from build123d import *

# Parameters (mm, degrees)
PAROI_DEPTH                    = 55
ESQUISSE11_W                   = 10
ESQUISSE11_H                   = 10
FIXATION_PAROI_BASE_DEPTH      = 3
ESQUISSE13_R                   = 1.5
TROU_FIXATION_PAROI_BASE_DEPTH = 4
EXTRUSION_BUMPER_REACH         = 108.066
ESQUISSE14_W                   = 172.132034356
ESQUISSE14_H                   = 30
BOSS_EXTRU_1_REACH             = 108.066
ESQUISSE15_W                   = 20
ESQUISSE15_H                   = 5
BOSS_EXTRU_2_DEPTH             = 35
ENL_V_MAT_EXTRU_1_REACH        = 108.066
ESQUISSE17_R                   = 2
ESQUISSE18_W                   = 10
ESQUISSE18_H                   = 10
ESQUISSE18_R                   = 1.5
BOSS_EXTRU_3_DEPTH             = 3
ESQUISSE20_W                   = 10
ESQUISSE20_H                   = 6
ESQUISSE20_W_2                 = 6
ESQUISSE20_H_2                 = 8
ENL_V_MAT_EXTRU_2_DEPTH        = 107.066017178
BOSS_EXTRU_4_DEPTH             = 5
BOSS_EXTRU_5_DEPTH             = 5
ENL_V_MAT_EXTRU_3_REACH        = 83.632
ESQUISSE25_R                   = 1.5
ESQUISSE35_R                   = 3
ENL_V_MAT_EXTRU_4_DEPTH        = 12
CONG_1_R                       = 5
CONG_2_R                       = 2


with BuildPart() as part:
    # Esquisse1 → paroi (new body)
    with BuildSketch(Plane.XY):
        with BuildLine():
            Line((0, 150), (0, 145))
            ThreePointArc((0, 145), (102.530483272, 102.530483272), (145, 0))
            Line((145, 0), (150, 0))
            ThreePointArc((150, 0), (106.066017178, 106.066017178), (0, 150))
        make_face()
    extrude(amount=PAROI_DEPTH)

    # Esquisse11 → fixation_paroi_base (add)
    with BuildSketch(Plane(origin=(0, 0, 0), x_dir=(-1, 0, 0), z_dir=(0, 0, -1))):
        with Locations((-140, 5)):
            Rectangle(ESQUISSE11_W, ESQUISSE11_H)
        with Locations((-5, 140)):
            Rectangle(ESQUISSE11_W, ESQUISSE11_H)
    extrude(amount=-FIXATION_PAROI_BASE_DEPTH)

    # Esquisse13 → trou_fixation_paroi_base (cut, through all)
    with BuildSketch(Plane.XY.offset(3)):
        with Locations((5, 140)):
            Circle(ESQUISSE13_R)
        with Locations((140, 5)):
            Circle(ESQUISSE13_R)
    extrude(amount=-TROU_FIXATION_PAROI_BASE_DEPTH, mode=Mode.SUBTRACT)

    # Esquisse14 → extrusion bumper (cut, up to next)
    with BuildSketch(Plane(origin=(75, 75, 0), x_dir=(-0.707106781, 0.707106781, 0), z_dir=(-0.707106781, -0.707106781, 0)), mode=Mode.PRIVATE) as extrusion_bumper_sk1:
        with Locations((0, -25)):
            Rectangle(ESQUISSE14_W, ESQUISSE14_H)
    extrusion_bumper_tool1 = extrude(extrusion_bumper_sk1.sketch, amount=-EXTRUSION_BUMPER_REACH, mode=Mode.PRIVATE) & part.part
    add(extrusion_bumper_tool1.solids().sort_by_distance((75, 75, 25))[0], mode=Mode.SUBTRACT)

    # Esquisse15 → Boss.-Extru.1 (add, up to next)
    with BuildSketch(Plane(origin=(75, 75, 0), x_dir=(-0.707106781, 0.707106781, 0), z_dir=(-0.707106781, -0.707106781, 0)), mode=Mode.PRIVATE) as boss_extru_1_sk1:
        with Locations((76.066017178, -42.5)):
            Rectangle(ESQUISSE15_W, ESQUISSE15_H)
    boss_extru_1_tool1 = extrude(boss_extru_1_sk1.sketch, amount=-BOSS_EXTRU_1_REACH, mode=Mode.PRIVATE) - part.part
    add(boss_extru_1_tool1.solids().sort_by_distance((21.213203, 128.786797, 42.5))[0])
    # Esquisse15 → Boss.-Extru.1 (add, up to next)
    with BuildSketch(Plane(origin=(75, 75, 0), x_dir=(-0.707106781, 0.707106781, 0), z_dir=(-0.707106781, -0.707106781, 0)), mode=Mode.PRIVATE) as boss_extru_1_sk2:
        with Locations((-76.066017178, -42.5)):
            Rectangle(ESQUISSE15_W, ESQUISSE15_H)
    boss_extru_1_tool2 = extrude(boss_extru_1_sk2.sketch, amount=-BOSS_EXTRU_1_REACH, mode=Mode.PRIVATE) - part.part
    add(boss_extru_1_tool2.solids().sort_by_distance((128.786797, 21.213203, 42.5))[0])
    # Esquisse15 → Boss.-Extru.1 (add, up to next)
    with BuildSketch(Plane(origin=(75, 75, 0), x_dir=(-0.707106781, 0.707106781, 0), z_dir=(-0.707106781, -0.707106781, 0)), mode=Mode.PRIVATE) as boss_extru_1_sk3:
        with Locations((76.066017178, -7.5)):
            Rectangle(ESQUISSE15_W, ESQUISSE15_H)
    boss_extru_1_tool3 = extrude(boss_extru_1_sk3.sketch, amount=-BOSS_EXTRU_1_REACH, mode=Mode.PRIVATE) - part.part
    add(boss_extru_1_tool3.solids().sort_by_distance((21.213203, 128.786797, 7.5))[0])
    # Esquisse15 → Boss.-Extru.1 (add, up to next)
    with BuildSketch(Plane(origin=(75, 75, 0), x_dir=(-0.707106781, 0.707106781, 0), z_dir=(-0.707106781, -0.707106781, 0)), mode=Mode.PRIVATE) as boss_extru_1_sk4:
        with Locations((-76.066017178, -7.5)):
            Rectangle(ESQUISSE15_W, ESQUISSE15_H)
    boss_extru_1_tool4 = extrude(boss_extru_1_sk4.sketch, amount=-BOSS_EXTRU_1_REACH, mode=Mode.PRIVATE) - part.part
    add(boss_extru_1_tool4.solids().sort_by_distance((128.786797, 21.213203, 7.5))[0])

    # Esquisse16 → Boss.-Extru.2 (add)
    with BuildSketch(Plane.XY.offset(45)):
        Polygon((135.857864376, 14.142135624), (121.715728753, 28.284271247), (125.251262658, 31.819805153), (139.393398282, 17.67766953), align=None)
        Polygon((28.284271247, 121.715728753), (14.142135624, 135.857864376), (17.67766953, 139.393398282), (31.819805153, 125.251262658), align=None)
    extrude(amount=-BOSS_EXTRU_2_DEPTH)

    # Esquisse17 → Enlèv. mat.-Extru.1 (cut, up to next)
    with BuildSketch(Plane(origin=(75, 75, 0), x_dir=(-0.707106781, 0.707106781, 0), z_dir=(-0.707106781, -0.707106781, 0)), mode=Mode.PRIVATE) as enl_v_mat_extru_1_sk1:
        with Locations((76.066017178, -25)):
            Circle(ESQUISSE17_R)
    enl_v_mat_extru_1_tool1 = extrude(enl_v_mat_extru_1_sk1.sketch, amount=-ENL_V_MAT_EXTRU_1_REACH, mode=Mode.PRIVATE) & part.part
    add(enl_v_mat_extru_1_tool1.solids().sort_by_distance((21.213203, 128.786797, 25))[0], mode=Mode.SUBTRACT)
    # Esquisse17 → Enlèv. mat.-Extru.1 (cut, up to next)
    with BuildSketch(Plane(origin=(75, 75, 0), x_dir=(-0.707106781, 0.707106781, 0), z_dir=(-0.707106781, -0.707106781, 0)), mode=Mode.PRIVATE) as enl_v_mat_extru_1_sk2:
        with Locations((-76.066017178, -25)):
            Circle(ESQUISSE17_R)
    enl_v_mat_extru_1_tool2 = extrude(enl_v_mat_extru_1_sk2.sketch, amount=-ENL_V_MAT_EXTRU_1_REACH, mode=Mode.PRIVATE) & part.part
    add(enl_v_mat_extru_1_tool2.solids().sort_by_distance((128.786797, 21.213203, 25))[0], mode=Mode.SUBTRACT)

    # Esquisse18 → Boss.-Extru.3 (add)
    with BuildSketch(Plane.XY.offset(55)):
        with Locations((5, 140)):
            Rectangle(ESQUISSE18_W, ESQUISSE18_H)
        with Locations((5, 140)):
            Circle(ESQUISSE18_R, mode=Mode.SUBTRACT)
        with Locations((140, 5)):
            Rectangle(ESQUISSE18_W, ESQUISSE18_H)
        with Locations((140, 5)):
            Circle(ESQUISSE18_R, mode=Mode.SUBTRACT)
    extrude(amount=-BOSS_EXTRU_3_DEPTH)

    # Esquisse20 → Enlèv. mat.-Extru.2 (cut, through all)
    with BuildSketch(Plane(origin=(75, 75, 0), x_dir=(-0.707106781, 0.707106781, 0), z_dir=(-0.707106781, -0.707106781, 0))):
        with Locations((76.066017178, -34)):
            Rectangle(ESQUISSE20_W, ESQUISSE20_H)
        with Locations((76.066017178, -16)):
            Rectangle(ESQUISSE20_W_2, ESQUISSE20_H_2)
        with Locations((-76.066017178, -34)):
            Rectangle(ESQUISSE20_W, ESQUISSE20_H)
        with Locations((-76.066017178, -16)):
            Rectangle(ESQUISSE20_W_2, ESQUISSE20_H_2)
    extrude(amount=-ENL_V_MAT_EXTRU_2_DEPTH, mode=Mode.SUBTRACT)

    # Esquisse21 → Boss.-Extru.4 (add)
    with BuildSketch(Plane.XY.offset(45)):
        Polygon((71.4177849, 130.81475452), (78.488852712, 123.743686708), (69.650017947, 114.904851943), (62.578950135, 121.975919755), align=None)
        Polygon((130.81475452, 71.4177849), (123.743686708, 78.488852712), (114.904851943, 69.650017947), (121.975919755, 62.578950135), align=None)
    extrude(amount=-BOSS_EXTRU_4_DEPTH)

    # Esquisse24 → Boss.-Extru.5 (add)
    with BuildSketch(Plane.XY.offset(10)):
        Polygon((62.578950135, 121.975919755), (71.065878403, 130.462848023), (78.136946215, 123.391780211), (69.650017947, 114.904851943), align=None)
        Polygon((121.975919755, 62.578950135), (130.462848023, 71.065878403), (123.391780211, 78.136946215), (114.904851943, 69.650017947), align=None)
    extrude(amount=-BOSS_EXTRU_5_DEPTH)

    # Esquisse25 → Enlèv. mat.-Extru.3 (cut, up to next)
    with BuildSketch(Plane(origin=(92.277434945, 92.277434945, 0), x_dir=(0, 0, 1), z_dir=(-0.707106781, -0.707106781, 0)), mode=Mode.PRIVATE) as enl_v_mat_extru_3_sk1:
        with Locations((42.5, 37.5)):
            Circle(ESQUISSE25_R)
    enl_v_mat_extru_3_tool1 = extrude(enl_v_mat_extru_3_sk1.sketch, amount=-ENL_V_MAT_EXTRU_3_REACH, mode=Mode.PRIVATE) & part.part
    add(enl_v_mat_extru_3_tool1.solids().sort_by_distance((65.760931, 118.793939, 42.5))[0], mode=Mode.SUBTRACT)
    # Esquisse25 → Enlèv. mat.-Extru.3 (cut, up to next)
    with BuildSketch(Plane(origin=(92.277434945, 92.277434945, 0), x_dir=(0, 0, 1), z_dir=(-0.707106781, -0.707106781, 0)), mode=Mode.PRIVATE) as enl_v_mat_extru_3_sk2:
        with Locations((42.5, -37.5)):
            Circle(ESQUISSE25_R)
    enl_v_mat_extru_3_tool2 = extrude(enl_v_mat_extru_3_sk2.sketch, amount=-ENL_V_MAT_EXTRU_3_REACH, mode=Mode.PRIVATE) & part.part
    add(enl_v_mat_extru_3_tool2.solids().sort_by_distance((118.793939, 65.760931, 42.5))[0], mode=Mode.SUBTRACT)
    # Esquisse25 → Enlèv. mat.-Extru.3 (cut, up to next)
    with BuildSketch(Plane(origin=(92.277434945, 92.277434945, 0), x_dir=(0, 0, 1), z_dir=(-0.707106781, -0.707106781, 0)), mode=Mode.PRIVATE) as enl_v_mat_extru_3_sk3:
        with Locations((7.5, 37.5)):
            Circle(ESQUISSE25_R)
    enl_v_mat_extru_3_tool3 = extrude(enl_v_mat_extru_3_sk3.sketch, amount=-ENL_V_MAT_EXTRU_3_REACH, mode=Mode.PRIVATE) & part.part
    add(enl_v_mat_extru_3_tool3.solids().sort_by_distance((65.760931, 118.793939, 7.5))[0], mode=Mode.SUBTRACT)
    # Esquisse25 → Enlèv. mat.-Extru.3 (cut, up to next)
    with BuildSketch(Plane(origin=(92.277434945, 92.277434945, 0), x_dir=(0, 0, 1), z_dir=(-0.707106781, -0.707106781, 0)), mode=Mode.PRIVATE) as enl_v_mat_extru_3_sk4:
        with Locations((7.5, -37.5)):
            Circle(ESQUISSE25_R)
    enl_v_mat_extru_3_tool4 = extrude(enl_v_mat_extru_3_sk4.sketch, amount=-ENL_V_MAT_EXTRU_3_REACH, mode=Mode.PRIVATE) & part.part
    add(enl_v_mat_extru_3_tool4.solids().sort_by_distance((118.793939, 65.760931, 7.5))[0], mode=Mode.SUBTRACT)

    # Esquisse35 → Enlèv. mat.-Extru.4 (cut)
    with BuildSketch(Plane(origin=(106.066017178, 106.066017178, 0), x_dir=(0, 0, 1), z_dir=(-0.707106781, -0.707106781, 0))):
        with Locations((42.5, -37.5)):
            Circle(ESQUISSE35_R)
        with Locations((42.5, 37.5)):
            Circle(ESQUISSE35_R)
        with Locations((7.5, -37.5)):
            Circle(ESQUISSE35_R)
        with Locations((7.5, 37.5)):
            Circle(ESQUISSE35_R)
    extrude(amount=ENL_V_MAT_EXTRU_4_DEPTH, mode=Mode.SUBTRACT)

    # Congé1
    cong_1_edges = [part.edges().sort_by_distance(p)[0] for p in [
        (77.375082971, 122.629916967, 42.5),
        (122.629916967, 77.375082971, 42.5),
        (77.375082971, 122.629916967, 7.5),
        (122.629916967, 77.375082971, 7.5),
    ]]
    fillet(cong_1_edges, radius=CONG_1_R)

    # Congé2
    cong_2_edges = [part.edges().sort_by_distance(p)[0] for p in [
        (68.436626134, 127.833595754, 42.5),
        (127.833595754, 68.436626134, 42.5),
        (68.436626134, 127.833595754, 7.5),
        (127.833595754, 68.436626134, 7.5),
    ]]
    fillet(cong_2_edges, radius=CONG_2_R)


solid = part.part
Work out the finished part from the listing and answer in its coordinate system (mm). A direction names the side the tool comes from. Round coordinates to 2 decimals unless told otherwise and drop trailing zeros. Loops run counter-clockwise (first coordinate to the right, second up) from the corner with the lowest first, then second, coordinate; pieces in that order, holes last. Notation, with made-up numbers: (56.5, -6) - (63.5, -6) arc R30 cw to (63.5, 26) - close; hole circle Ø1 at (-37.75, -1.5). An arc over 180 degrees is marked (long way). One line per item, written item: value.
Q1. Straight lines are drawn through the part: probe 1 along X at (y, z) = (14.5, 16); probe 2 along Y at (x, z) = (5, 52.9); probe 3 along Y at (x, z) = (64, 7.5). For each, find the intervals that lie inside material, in ascending order.
Check values:
probe 1: 135.5 to 136.22, 144.27 to 149.3
probe 2: 135 to 138.5, 141.5 to 149.92
probe 3: 120.55 to 123.4, 130.11 to 135.66
Q2. Each of these flat-tipped pins is pushed along its axis until it touches: pin 1 Ø8 at (y, z) = (115.5, 44) entering from +X; pin 2 Ø6.5 at (x, y) = (133, 22) entering from -Z; pin 3 Ø12 at (y, z) = (25.5, 15) entering from -X; pin 4 Ø2.5 at (x, y) = (140, 5) entering from -Z. Where does it stop, or does it pass through?
Check values:
pin 1: x = 100.34
pin 2: z = 5
pin 3: x = 121.72
pin 4: through
Q3. Find section B-B on x = 52. Give the vertices of the cut face in (y, z), and give its area (3 significant figures).
Check values:
outline: (135.36, 0) - (140.7, 0) - (140.7, 10) - (135.36, 10) - close; (135.36, 40) - (140.7, 40) - (140.7, 55) - (135.36, 55) - close
area: 134 mm2
Q4. For faces 4 (the flat face through (117.368, 72.114, 7.535)), 5 (the flat face through (132.651, 20.835, 16.056)), 6 (the flat face through (130.65, 26.42, 25.21)), 7 (the flat face through (71.98, 123.18, 8.58)), determine the directions among +Z, -Z, +X, -X, +Y, -Y from which every point of the face is accessible in a straight line to the end or side of a thin tool.
Check values:
face 4: +Z, -Z, -X
face 5: -X, +Y
face 6: +Y
face 7: none
Q5. Find section A-A on y = 54. Give the vertices of the cut face in (x, z), and give its area (3 significant figures).
Check values:
outline: (134.57, 0) - (139.94, 0) - (139.94, 10) - (134.57, 10) - close; (134.57, 40) - (139.94, 40) - (139.94, 55) - (134.57, 55) - close
area: 134 mm2
Q6. The mould has two halves that part along Z. Classify faces 1 (the flat face through (102.4, 103.1, 55)), 2 (the flat face through (131, 23, 12)), 3 (the cylindrical face through (77.5, 121.2, 7.5)): +Z half, -Z half, draft (parallel to the pull), parting line (faces both ways), or undercut.
Check values:
face 1: +Z half
face 2: undercut
face 3: draft
